Autodesk Inventor part; units mm, degrees
ref_plane "YZ Plane" through (0, 0, 0) normal (1, 0, 0) x (0, 1, 0)
ref_plane "XZ Plane" through (0, 0, 0) normal (0, 1, 0) x (-1, 0, 0)
ref_plane "XY Plane" through (0, 0, 0) normal (0, 0, 1) x (1, 0, 0)
sketch "Sketch1" plane through (0, 0, 0) normal (0, 0, 1) x (1, 0, 0)
  circle A0 centre (0, 0) radius 45.72
  dimension "d0" = 91.44
extrude "Extrusion1" add sketch "Sketch1" along normal blind 15.24
sketch "Sketch2" plane through (0, 0, 15.24) normal (0, 0, 1) x (1, 0, 0)
  circle A0 centre (0, 0) radius 17.78
  dimension "d3" = 35.56
extrude "Extrusion2" add sketch "Sketch2" along normal blind 33.02
sketch "Sketch3" plane through (0, 0, 48.26) normal (0, 0, 1) x (1, 0, 0)
  line L0 (4.0695, 7.0485) -> (8.1389, 0)
  line L1 (8.1389, 0) -> (4.0695, -7.0485)
  line L2 (4.0695, -7.0485) -> (-4.0695, -7.0485)
  line L3 (-4.0695, -7.0485) -> (-8.1389, 0)
  line L4 (-8.1389, 0) -> (-4.0695, 7.0485)
  line L5 (-4.0695, 7.0485) -> (4.0695, 7.0485)
  point P0 (0, 0)
  point P1 (0, 0)
  dimension "d6" = 14.097
extrude "Extrusion3" add sketch "Sketch3" along normal blind 8.382
sketch "Sketch4" plane through (0, 0, 56.642) normal (0, 0, 1) x (1, 0, 0)
  circle A0 centre (0, 0) radius 7.112
  dimension "d9" = 14.224
extrude "Extrusion4" add sketch "Sketch4" along normal blind 25.4
sketch "Sketch5" plane through (0, 0, 82.042) normal (0, 0, 1) x (1, 0, 0)
  circle A0 centre (0, 0) radius 2.413
  dimension "d12" = 4.826
extrude "Extrusion5" cut sketch "Sketch5" against normal up to surface (25.4 mm away)
sketch "Sketch6" plane through (0, 0, 0) normal (0, 0, -1) x (-1, 0, 0)
  circle A0 centre (0, 0) radius 45.72
  circle A1 centre (0, 0) radius 25.4
  dimension "d15" = 50.8
extrude "Extrusion6" cut sketch "Sketch6" against normal blind 5.08
sketch "Sketch7" plane through (0, 0, 0) normal (0, 0, -1) x (-1, 0, 0)
  circle A0 centre (0, 0) radius 17.145
  dimension "d19" = 34.29
extrude "Extrusion7" cut sketch "Sketch7" against normal blind 15.24
fillet "Fillet1" radius 3.175 3 edges at (-45.72, 0, 5.08) (25.4, 0, 5.08) (25.4, 0, 0)
sketch "Sketch8" plane through (0, 0, 15.24) normal (0, 0, -1) x (-1, 0, 0)
  line L0 (8.1389, 0) -> (4.0695, 7.0485)
  line L1 (4.0695, -7.0485) -> (8.1389, 0)
  line L2 (-4.0695, -7.0485) -> (4.0695, -7.0485)
  line L3 (-8.1389, 0) -> (-4.0695, -7.0485)
  line L4 (-4.0695, 7.0485) -> (-8.1389, 0)
  line L5 (4.0695, 7.0485) -> (-4.0695, 7.0485)
  line L6 (4.0695, 7.0485) -> (8.1389, 0)
  line L7 (8.1389, 0) -> (4.0695, -7.0485)
  line L8 (4.0695, -7.0485) -> (-4.0695, -7.0485)
  line L9 (-4.0695, -7.0485) -> (-8.1389, 0)
  line L10 (-8.1389, 0) -> (-4.0695, 7.0485)
  line L11 (-4.0695, 7.0485) -> (4.0695, 7.0485)
  point P0 (0, 0)
  point P1 (0, 0)
extrude "Extrusion8" cut sketch "Sketch8" against normal blind 29.845
sketch "Sketch9" plane through (0, 0, 15.24) normal (0, 0, 1) x (1, 0, 0)
  circle A0 centre (31.75, 0) radius 6.985
  circle A1 centre (0, 0) radius 45.72
  line L0 (31.75, 0) -> (45.72, 0) construction
  line L1 (0, 0) -> (31.75, 0) construction
  dimension "d24" = 13.97
  dimension "d25" = 13.97
extrude "Extrusion9" cut sketch "Sketch9" against normal blind 5.08 contours A0
pattern_circular "Circular Pattern1" count 3 over 360 about axis through (0, 0, 15.24) along (0, 0, 1) of "Extrusion9"
properties part number "Cutter"
The model under review builds one solid part; all positions refer to its coordinate system, in mm. A direction names the side the tool comes from. Round coordinates to 2 decimals unless told otherwise and drop trailing zeros. Loops run counter-clockwise (first coordinate to the right, second up) from the corner with the lowest first, then second, coordinate; pieces in that order, holes last. Notation, with made-up numbers: (31, -40) -> (72, -40) arc R15 ccw to (72, -20) -> close; hole circle Ø6 at (81, 0). An arc over 180 degrees is marked (long way). Write item = value, one per line. Start each with the question number.
Item 1: Take a section at C-C on z = 73. Give the boundary of the cut face in (x, y), plus the area to 3 significant figures.
Item 2: Take a section at A-A on z = 35. Give the boundary of the cut face in (x, y), plus the area to 3 significant figures.
Item 3: Insertion check: pin 1 (11 mm diameter, centred on x = 34, y = 3, fed in from +Z); pin 2 (9 mm diameter, centred on x = 0.5, z = 54, fed in from +Y); pin 3 (11 mm diameter, centred on x = -15.88, y = 27.5, fed in from -Z). Each pin has a flat end and moves straight along its axis. Give the tip position at first contact, or say it passes through.
Item 4: For faces 1 (the flat face through (3.6, 6.4, 56.642)), 2 (the flat face through (6.133, -3.475, 29.954)), 3 (the flat face through (-3.6, 6.4, 56.642)), 4 (the cylindrical face through (-21.02, 32.22, 12.74)), 5 (the flat face through (3.8, -6.3, 56.642)), list the 3-axis set-ups (+Z, -Z, +X, -X, +Y, -Y) from which the entire face can be reached by the end or side of a thin tool; tool diameter is ignored.
Item 5: Mouldability with a two-part tool opening along Y and no side actions: class faces 6 (the cylindrical face through (-21.418, -31.747, 12.736)), 7 (the flat face through (0, -7.048, 52)), 8 (the cylindrical face through (-1.542, 6.943, 69.164)), 9 (the flat face through (20, 1, 15.24)) as released by +Y, released by -Y, zero draft, split by the parting line, or undercut.
Item 6: Take a section at B-B on z = 13.5. Count the separate pieces of the cut face and the enclosed holes in it, plus the area to 3 significant figures.
Item 7: To check wall thickness, follow L1, parallel to Z at x = 33, y = 6; L2, parallel to Z at x = 15.5, y = 0.5; L3, parallel to X at y = 10, z = 6. State the ranges of each line that lie inside material, in increasing order.
Result:
q1.outline = circle Ø14.22 at (0, 0); hole circle Ø4.83 at (0, 0)
q1.area = 141 mm²
q2.outline = circle Ø35.56 at (0, 0); hole (-8.14, 0) -> (-4.07, -7.05) -> (4.07, -7.05) -> (8.14, 0) -> (4.07, 7.05) -> (-4.07, 7.05) -> close
q2.area = 821 mm²
q3.pin_1 = 15.24
q3.pin_2 = 7.11
q3.pin_3 = 4.07
q4.face_1 = +Z, +X, +Y
q4.face_2 = -Z
q4.face_3 = +Z, -X, +Y
q4.face_4 = +Z
q4.face_5 = +Z, +X, -Y
q5.face_6 = undercut
q5.face_7 = released by -Y
q5.face_8 = split by the parting line
q5.face_9 = zero draft
q6.separate_pieces = 1
q6.enclosed_holes = 4
q6.area = 5,180 mm²
q7.L1 = 5.08 to 10.16
q7.L2 = 15.24 to 48.26
q7.L3 = -43.65 to -13.93, 13.93 to 43.65
